Geometry: final body of the model. Coordinates: model frame, mm. Face numbers are marked on the shaded views. A direction names the side the tool comes from. Round coordinates to 2 decimals unless told otherwise and drop trailing zeros. Loops run counter-clockwise (first coordinate to the right, second up) from the corner with the lowest first, then second, coordinate; pieces in that order, holes last. Notation, with made-up numbers: (81.25, 69.25) - (91.25, 69.25) arc R13 cw to (91.25, 94.25) - close; hole circle Ø8 at (29.5, -10). An arc over 180 degrees is marked (long way). Write item = value, one per line. Start each with the question number.
Item 1: Section A-A (x = 38.5). Return loops of the section in (y, z), plus the area to 3 significant figures.
Item 2: Access query for the marked faces 1 and 2. Directions: +Z, -Z, +X, -X, +Y, -Y. A direction counts if a zero-diameter tool reaches every point of the face in a straight line with its end or side. Return the directions, or none.
Item 3: Section C-C (y = 6). Return loops of the section in (x, z).
Item 4: Line query: line 1 (Z direction, x = 35.2, y = 7.75); line 2 (X direction, y = 3, z = -9); line 3 (Y direction, x = -14, z = -0.5). Output: solid intervals per line, ascending. Write a range as from..to.
Item 5: Section B-B (x = -17). Return loops of the section in (y, z).
Item 6: First-contact query: pin 1 (10 mm diameter, centred on x = -23.5, z = -6.5, fed in from +Y); pin 2 (1.5 mm diameter, centred on x = 14, z = -7.5, fed in from -Y); pin 3 (2 mm diameter, centred on x = 19.5, y = -17.5, fed in from +Z). Flat tips, straight axial feed; report the tip coordinate or a pass-through.
Item 7: Draft query along X for the marked faces 3, 4 and 5. Return one class per face: pulls with the +X half, pulls with the -X half, needs draft (parallel to the pull), parting line crosses it, or undercut.
Item 8: Section D-D (z = 31). Return loops of the section in (x, y).
from build123d import *

# Parameters (mm, degrees)
SKETCH1_W           = 80
SKETCH1_H           = 60
BOSS_EXTRUDE1_DEPTH = 10
SKETCH2_R           = 5.5
CUT_EXTRUDE1_DEPTH  = 58.879184514
SKETCH3_W           = 79.999469754
SKETCH3_H           = 3
BOSS_EXTRUDE2_DEPTH = 30


with BuildPart() as part:
    # Sketch1 → Boss-Extrude1 (new body)
    with BuildSketch(Plane(origin=(0, 0, 0), x_dir=(1, 0, 0), z_dir=(0, 1, 0))):
        with Locations((5, -5)):
            Rectangle(SKETCH1_W, SKETCH1_H)
    extrude(amount=BOSS_EXTRUDE1_DEPTH)

    # Sketch2 → Cut-Extrude1 (cut, through all)
    with BuildSketch(Plane(origin=(0, 10, 0), x_dir=(1, 0, 0), z_dir=(0, 1, 0))):
        with Locations(Location((-25.20025306, 5.49130346, 0), (0, 0, 270))):
            Circle(SKETCH2_R)
        with Locations(Location((35.2, 5.49130346, 0), (0, 0, 90))):
            Circle(SKETCH2_R)
    extrude(amount=-CUT_EXTRUDE1_DEPTH, mode=Mode.SUBTRACT)

    # Sketch3 → Boss-Extrude2 (add)
    with BuildSketch(Plane.XZ):
        with Locations((5.000265123, -23.5)):
            Rectangle(SKETCH3_W, SKETCH3_H)
    extrude(amount=BOSS_EXTRUDE2_DEPTH)


solid = part.part
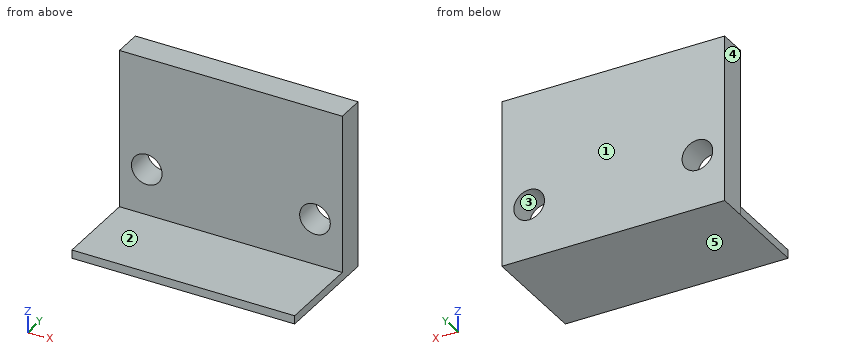
Taken from the geometry:
q1.outline = (-30, -25) - (10, -25) - (10, -9.89) - (0, -9.89) - (0, -22) - (-30, -22) - close; (0, -1.09) - (10, -1.09) - (10, 35) - (0, 35) - close
q1.area = 602 mm^2
q2.face_1 = +Z, -Z, +X, -X, +Y
q2.face_2 = +Z, +X, -X, -Y
q3.outline = (-35, -25) - (45, -25) - (45, 35) - (-35, 35) - close; hole circle Ø11 at (-25.2, -5.49); hole circle Ø11 at (35.2, -5.49)
q4.line_1 = -25..-10.99, 0.01..35
q4.line_2 = -35..-29.44, -20.96..30.96, 39.44..45
q4.line_3 = 0..10
q5.outline = (-30, -25) - (10, -25) - (10, 35) - (0, 35) - (0, -22) - (-30, -22) - close
q6.pin_1 = 10
q6.pin_2 = 0
q6.pin_3 = -22
q7.face_3 = undercut
q7.face_4 = pulls with the -X half
q7.face_5 = needs draft
q8.outline = (-35, 0) - (45, 0) - (45, 10) - (-35, 10) - close
